The model under review builds one solid part; all positions refer to its coordinate system, in mm. A direction names the side the tool comes from. Coordinates: 2 decimals unless noted, no trailing zeros. Order: outer loops, then holes, each group sorted by start corner. A loop starts at its lowest first (then second) coordinate and runs counter-clockwise, first axis right, second up.
from build123d import *

# Parameters (mm, degrees)
EXTRUDE_1_DEPTH     = 5
EXTRUDE_2_DEPTH     = 5
EXTRUDE_3_DEPTH     = 5
EXTRUDE_4_DEPTH     = 5
EXTRUDE_5_DEPTH     = 50
CUT_EXTRUDE_1_DEPTH = 30
FILLET_1_R          = 5
SKETCH_6_R          = 1.6499999999999952
CUT_EXTRUDE_2_DEPTH = 60
FILLET_2_R          = 5
CHAMFER_1_SIZE      = 5
FILLET_3_R          = 5
FILLET_4_R          = 5


# Some blends are built 0.0001 mm under size
with BuildPart() as part:
    # 스케치1 → 보스-돌출1 (new body)
    with BuildSketch(Plane.XY):
        Polygon((-10.000000000000016, 100), (10.000000000000016, 100), (10.000000000000002, 0), (-10.000000000000002, 0), align=None)
    extrude(amount=EXTRUDE_1_DEPTH)

    # 스케치2 → 보스-돌출2 (add)
    with BuildSketch(Plane(origin=(0, 0, 0), x_dir=(1, 0, 0), z_dir=(0, 1, 0))):
        Polygon((-10.000000000000002, 0), (10.000000000000002, 0), (10.000000000000005, -25.2), (-9.999999999999998, -25.2), align=None)
    extrude(amount=-EXTRUDE_2_DEPTH)

    # 스케치3 → 보스-돌출3 (add)
    with BuildSketch(Plane.XY.offset(25.2)):
        Polygon((-50, 0), (50, 0), (50, -19.999999999999986), (-50, -20), align=None)
    extrude(amount=-EXTRUDE_3_DEPTH)

    # 스케치4 → 보스-돌출4 (add)
    with BuildSketch(Plane.XY.offset(25.2)):
        Polygon((50, -19.999999999999996), (35, -19.999999999999996), (34.99999999999999, 100.00000000000001), (49.999999999999986, 100.00000000000001), align=None)
        Polygon((-50.000000000000014, 100), (-35.000000000000014, 100), (-35, -19.999999999999996), (-50, -19.999999999999996), align=None)
    extrude(amount=EXTRUDE_4_DEPTH)

    # 스케치5 → 보스-돌출5 (add, symmetric)
    with BuildSketch(Plane(origin=(0, 0, 0), x_dir=(0, 0, -1), z_dir=(1, 0, 0))):
        Polygon((-20.2, -20), (-143.76355340335743, -59.26033642854078), (-147.01597593744285, -49.02402869306782), (-20.2, -8.730287191761477), align=None)
    extrude(amount=EXTRUDE_5_DEPTH, both=True)

    # 스케치5<3> → 컷-돌출1 (cut, symmetric)
    with BuildSketch(Plane(origin=(0, 0, 0), x_dir=(0, 0, -1), z_dir=(1, 0, 0))):
        Polygon((-20.2, -20), (-143.76355340335743, -59.26033642854078), (-147.01597593744285, -49.02402869306782), (-20.2, -8.730287191761477), align=None)
    extrude(amount=CUT_EXTRUDE_1_DEPTH, both=True, mode=Mode.SUBTRACT)

    # 필렛1
    fillet_1_edges = [part.edges().sort_by_distance(p)[0] for p in [
        (42.5, -11.90762673462655, 30.199999999999996),
        (-42.5, -11.90762673462655, 30.199999999999996),
    ]]
    fillet(fillet_1_edges, radius=FILLET_1_R)

    # 스케치6 → 컷-돌출2 (cut)
    with BuildSketch(Plane.XY.offset(30.200000000000003)):
        with Locations((-42.500000000000014, 90.00000000000001)):
            Circle(SKETCH_6_R)
        with Locations(Location((42.500000000000014, 90.00000000000001, 0), (0, 0, 180))):
            Circle(SKETCH_6_R)
    extrude(amount=-CUT_EXTRUDE_2_DEPTH, mode=Mode.SUBTRACT)

    # 필렛2
    fillet_2_edges = [part.edges().sort_by_distance(p)[0] for p in [
        (-40, -59.26033642854078, 143.76355340335743),
        (-40, -49.02402869306782, 147.01597593744285),
        (40, -49.02402869306782, 147.01597593744285),
        (40, -59.26033642854078, 143.76355340335743),
    ]]
    fillet(fillet_2_edges, radius=FILLET_2_R)

    # 모따기1
    chamfer_1_edges = [part.edges().sort_by_distance(p)[0] for p in [
        (-35, -5.159478481597006, 25.2),
        (35, -5.159478481597006, 25.2),
    ]]
    chamfer(chamfer_1_edges, length=CHAMFER_1_SIZE - 0.0001)  # a hair under: the kernel refuses the full size

    # 필렛3
    fillet_3_edges = [part.edges().sort_by_distance(p)[0] for p in [
        (30, -9.52462207747773, 22.699999999999974),
        (-30, -9.52462207747773, 22.699999999999974),
    ]]
    fillet(fillet_3_edges, radius=FILLET_3_R)

    # 필렛4
    # the kernel refuses this fillet: 5 mm, written as the material it adds along each edge
    with BuildSketch(Plane(origin=(10, -5, 20.2), x_dir=(1, -1.4e-16, 0), z_dir=(1.4e-16, 1, 0)), Plane(origin=(-10, 0, 20.2), x_dir=(-1, -1.4e-16, 0), z_dir=(1.4e-16, -1, 0))) as fillet_4_piece_1:
        with BuildLine():
            CenterArc((FILLET_4_R, FILLET_4_R), FILLET_4_R, 180, 90)
            Line((0, FILLET_4_R), (-FILLET_4_R * 0.02, FILLET_4_R))
            Line((-FILLET_4_R * 0.02, FILLET_4_R), (-FILLET_4_R * 0.02, -FILLET_4_R * 0.02))
            Line((-FILLET_4_R * 0.02, -FILLET_4_R * 0.02), (FILLET_4_R, -FILLET_4_R * 0.02))
            Line((FILLET_4_R, -FILLET_4_R * 0.02), (FILLET_4_R, 0))
        make_face()
    extrude(amount=5)
    with BuildSketch(Plane(origin=(-10.000000000000004, -5, 20.2), x_dir=(0, -1, 0), z_dir=(1, 0, 0))) as fillet_4_piece_2:
        with BuildLine():
            CenterArc((5, 4.8360965028207445), FILLET_4_R, 180, 75.28906399659809)
            Line((0, 4.8360965028207445), (-0.09999999999999964, 4.8360965028207445))
            Line((-0.09999999999999964, 4.8360965028207445), (-0.09999999999999964, 0))
            Line((-0.09999999999999964, 0), (0, -0.10000000000000142))
            ThreePointArc((0, -0.10000000000000142), (1.8651435958807383, -0.10000000000000142), (3.704892935596707, -0.0967219300564146))
            Line((3.704892935596707, -0.0967219300564146), (3.7302871917614766, 0))
        make_face()
    extrude(amount=20.000000000000007)
    with BuildSketch(Plane(origin=(-10.000000000000004, -5, 20.2), x_dir=(0, -1, 0), z_dir=(1, 0, 0))) as fillet_4_piece_3a_section:
        with BuildLine():
            CenterArc((5, 4.8360965028207445), FILLET_4_R, 180, 75.28906399659809)
            Line((0, 4.8360965028207445), (-0.09999999999999964, 4.8360965028207445))
            Line((-0.09999999999999964, 4.8360965028207445), (-0.09999999999999964, 0))
            Line((-0.09999999999999964, 0), (0, -0.10000000000000142))
            ThreePointArc((0, -0.10000000000000142), (1.8651435958807383, -0.10000000000000142), (3.704892935596707, -0.0967219300564146))
            Line((3.704892935596707, -0.0967219300564146), (3.7302871917614766, 0))
        make_face()
    fillet_4_piece_3a = extrude(amount=32.09024125705187, mode=Mode.PRIVATE)
    fillet_4_piece_3a = split(fillet_4_piece_3a, bisect_by=Plane(origin=(10.000000000000004, -5.000000000000003, 20.2), z_dir=(1, -1.4e-16, 0)), keep=Keep.TOP, mode=Mode.PRIVATE)
    with BuildSketch(Plane(origin=(9.999999999999998, -17.5, 20.2), x_dir=(1, -1.4e-16, 0), z_dir=(1.4e-16, 1, 0))) as fillet_4_piece_3b_section:
        with BuildLine():
            CenterArc((FILLET_4_R, FILLET_4_R), FILLET_4_R, 180, 90)
            Line((0, FILLET_4_R), (-FILLET_4_R * 0.02, FILLET_4_R))
            Line((-FILLET_4_R * 0.02, FILLET_4_R), (-FILLET_4_R * 0.02, -FILLET_4_R * 0.02))
            Line((-FILLET_4_R * 0.02, -FILLET_4_R * 0.02), (FILLET_4_R, -FILLET_4_R * 0.02))
            Line((FILLET_4_R, -FILLET_4_R * 0.02), (FILLET_4_R, 0))
        make_face()
    fillet_4_piece_3b = extrude(amount=17.5, mode=Mode.PRIVATE)
    fillet_4_piece_3b = split(fillet_4_piece_3b, bisect_by=Plane(origin=(9.999999999999998, -9.534448385301843, 22.730926212611323), z_dir=(0, 0.9530490272330943, 0.3028160360516808)), keep=Keep.TOP, mode=Mode.PRIVATE)
    fillet_4_piece_3b = split(fillet_4_piece_3b, bisect_by=Plane(origin=(9.999999999999998, -5, 20.2), z_dir=(0, -1, 0)), keep=Keep.TOP, mode=Mode.PRIVATE)
    fillet_4_piece_3 = fillet_4_piece_3a & fillet_4_piece_3b
    add(fillet_4_piece_3)
    with BuildSketch(Plane(origin=(-10, 0, 20.2), x_dir=(-1, -1.4e-16, 0), z_dir=(1.4e-16, -1, 0))) as fillet_4_piece_4a_section:
        with BuildLine():
            CenterArc((FILLET_4_R, FILLET_4_R), FILLET_4_R, 180, 90)
            Line((0, FILLET_4_R), (-FILLET_4_R * 0.02, FILLET_4_R))
            Line((-FILLET_4_R * 0.02, FILLET_4_R), (-FILLET_4_R * 0.02, -FILLET_4_R * 0.02))
            Line((-FILLET_4_R * 0.02, -FILLET_4_R * 0.02), (FILLET_4_R, -FILLET_4_R * 0.02))
            Line((FILLET_4_R, -FILLET_4_R * 0.02), (FILLET_4_R, 0))
        make_face()
    fillet_4_piece_4a = extrude(amount=17.5, mode=Mode.PRIVATE)
    fillet_4_piece_4a = split(fillet_4_piece_4a, bisect_by=Plane(origin=(-10, -7.929741230725918, 17.680451962292693), z_dir=(0, 0.9530490272330943, 0.3028160360516808)), keep=Keep.TOP, mode=Mode.PRIVATE)
    fillet_4_piece_4a = split(fillet_4_piece_4a, bisect_by=Plane(origin=(-10, -5, 20.2), z_dir=(0, -1, 0)), keep=Keep.TOP, mode=Mode.PRIVATE)
    with BuildSketch(Plane(origin=(-22.090241257051865, -5, 20.2), x_dir=(0, -1, 0), z_dir=(1, 0, 0))) as fillet_4_piece_4b_section:
        with BuildLine():
            CenterArc((5, 4.8360965028207445), FILLET_4_R, 180, 75.28906399659809)
            Line((0, 4.8360965028207445), (-0.09999999999999964, 4.8360965028207445))
            Line((-0.09999999999999964, 4.8360965028207445), (-0.09999999999999964, 0))
            Line((-0.09999999999999964, 0), (0, -0.10000000000000142))
            ThreePointArc((0, -0.10000000000000142), (1.8651435958807383, -0.10000000000000142), (3.704892935596707, -0.0967219300564146))
            Line((3.704892935596707, -0.0967219300564146), (3.7302871917614766, 0))
        make_face()
    fillet_4_piece_4b = extrude(amount=32.09024125705187, mode=Mode.PRIVATE)
    fillet_4_piece_4b = split(fillet_4_piece_4b, bisect_by=Plane(origin=(-10.000000000000002, -4.999999999999998, 20.2), z_dir=(-1, -1.4e-16, 0)), keep=Keep.TOP, mode=Mode.PRIVATE)
    fillet_4_piece_4 = fillet_4_piece_4a & fillet_4_piece_4b
    add(fillet_4_piece_4)


solid = part.part
(1) Consider section C-C (x = 4). Give the boundary of the cut face in (y, z).
(2) Consider section A-A (y = 23). Give the boundary of the cut face in (x, z), then the cut area to 3 significant figures.
(3) Tool access review of faces 1 (the face through (32.5, -6, 27.7)), 2 (the face through (43, 51, 25.2)), 3 (the face through (10, 44, 2)): name each direction out of +Z, -Z, +X, -X, +Y, -Y from which nothing blocks a thin tool from reaching the whole face with its end or side.
(4) Wall thickness on line 1 (Z direction, x = -40.5, y = -2.5); line 2 (Y direction, x = -42.5, z = 29); line 3 (Z direction, x = 40, y = 33): over which ranges is each line inside the solid? List them lowest first.
(5) Insertion check: pin 1 Ø12.5 at (x, z) = (18, 17.5) entering from +Y; pin 2 Ø4.5 at (x, y) = (-42.5, 27.5) entering from +Z; pin 3 Ø16.5 at (y, z) = (33, 6) entering from +X. Each pin has a flat end and moves straight along its axis. Give the tip position at first contact, or say it passes through.
(6) Consider section B-B (z = 132). Give the boundary of the cut face in (x, y).
(7) The part is to be moulded in two halves that separate along X. For faces 4 (the face through (50, -25, 64)), 5 (the face through (0.35, -9.536, 22.735)), 6 (the face through (28.57, -11.18, 22.96)), 7 (the face through (43, 47, 30.2)), say which applies: +X half, -X half, draft (parallel to the pull), parting line (faces both ways), or undercut.
(8) Consider section D-D (y = -45). Give the boundary of the cut face in (x, z).
Findings:
1. outline: (-10.32, 25.2) - (-8.73, 20.2) arc R5 cw to (-5, 15.36) - (-5, 0) - (100, 0) - (100, 5) - (0, 5) - (0, 25.2) - close
2. outline: (-50, 25.2) - (-35, 25.2) - (-35, 30.2) - (-50, 30.2) - close; (-10, 0) - (10, 0) - (10, 5) - (-10, 5) - close; (35, 25.2) - (50, 25.2) - (50, 30.2) - (35, 30.2) - close
2. area: 250 mm2
3. face 1: +Z, +Y
3. face 2: -Z, +X, -X, +Y
3. face 3: -Z, +X, +Y, -Y
4. line 1: z = 20.2 to 30.2
4. line 2: y = -22.8 to 88.35, 91.65 to 100
4. line 3: z = 25.2 to 30.2
5. pin 1: stops at y = 0
5. pin 2: stops at z = 30.2
5. pin 3: stops at x = 10
6. outline: (-50, -55.52) - (-30, -55.52) - (-30, -44.25) - (-50, -44.25) - close; (30, -55.52) - (50, -55.52) - (50, -44.25) - (30, -44.25) - close
7. face 4: +X half
7. face 5: undercut
7. face 6: undercut
7. face 7: draft
8. outline: (-50, 98.88) - (-30, 98.88) - (-30, 134.35) - (-50, 134.35) - close; (30, 98.88) - (50, 98.88) - (50, 134.35) - (30, 134.35) - close
